Design review of the part shown in the three views and the two pictorial views. Dimensions are in mm from the part's minimum x, y and z. Round coordinates to 2 decimals unless told otherwise and drop trailing zeros. Loops run counter-clockwise (first coordinate to the right, second up) from the corner with the lowest first, then second, coordinate; pieces in that order, holes last. Notation, with made-up numbers: (31.5, 25) -> (72.5, 25) arc R26 cw to (72.5, 40) -> close; hole circle Ø8 at (77.25, 44.25). An arc over 180 degrees is marked (long way). Use a Markdown table: item, result. Add a question column.
1) Consider section A-A on x = 38.1. Give the boundary of the cut face in (y, z).
2) Consider section C-C on y = 27. Give the boundary of the cut face in (x, z).
3) Wall thickness on probe 1 along Y at (x, z) = (38, 17); probe 2 along X at (y, z) = (41.5, 34.5) (1 decimal); probe 3 along X at (y, z) = (34, 33): over which ranges is each line inside the solid? List them lowest first.
4) Insertion check: pin 1 (2 mm diameter, centred on x = 20, z = 28.5, fed in from +Y) (1 decimal); pin 2 (3 mm diameter, centred on y = 41, z = 41.5, fed in from -X) (1 decimal); pin 3 (5 mm diameter, centred on y = 9, z = 27.5, fed in from +X); pin 4 (7.5 mm diameter, centred on x = 38.1, y = 36.75, fed in from +Z). Each pin has a flat end and moves straight along its axis. Give the tip position at first contact, or say it passes through.
5) Consider section B-B on z = 28. Give the boundary of the cut face in (x, y), plus the area to 3 significant figures.
6) Mouldability with a two-part tool opening along X and no side actions: class the marked faces 1, 2 and 3 as released by +X, released by -X, zero draft, split by the parting line, or undercut.
7) Consider section D-D on x = 54.5. Give the boundary of the cut face in (y, z) (1 decimal).
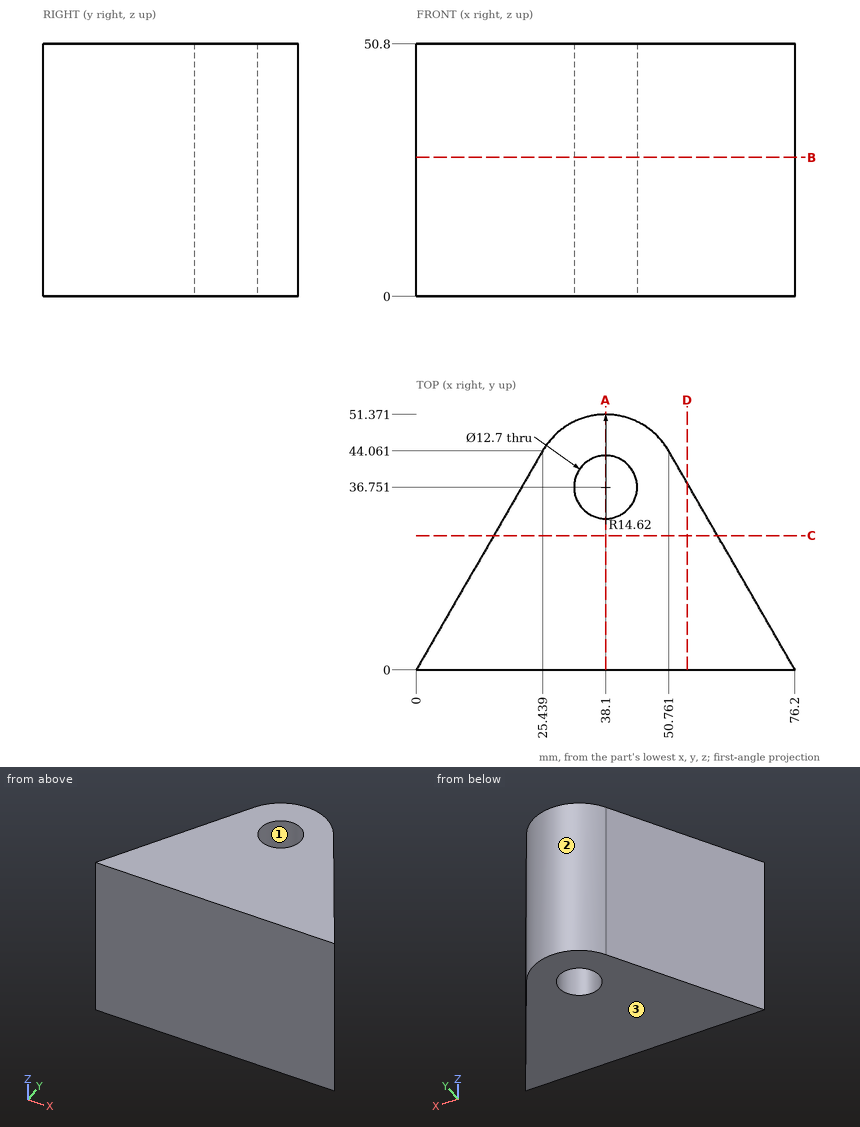
Result set:
| question | item | result |
|---|---|---|
| 1 | outline | (0, 0) -> (30.4, 0) -> (30.4, 50.8) -> (0, 50.8) -> close; (43.1, 0) -> (51.37, 0) -> (51.37, 50.8) -> (43.1, 50.8) -> close |
| 2 | outline | (15.59, 0) -> (60.61, 0) -> (60.61, 50.8) -> (15.59, 50.8) -> close |
| 3 | probe 1 | 0 to 30.4, 43.1 to 51.37 |
| 3 | probe 2 | 24 to 33.9, 42.3 to 52.2 |
| 3 | probe 3 | 19.63 to 32.38, 43.82 to 56.57 |
| 4 | pin 1 | y = 36.4 |
| 4 | pin 2 | x = 22.8 |
| 4 | pin 3 | x = 72.45 |
| 4 | pin 4 | through |
| 5 | outline | (0, 0) -> (76.2, 0) -> (50.76, 44.06) arc R14.62 ccw to (25.44, 44.06) -> close; hole circle Ø12.7 at (38.1, 36.75) |
| 5 | area | 2,240 mm2 |
| 6 | face 1 | undercut |
| 6 | face 2 | split by the parting line |
| 6 | face 3 | zero draft |
| 7 | outline | (0, 0) -> (37.6, 0) -> (37.6, 50.8) -> (0, 50.8) -> close |
